Input: part model. Units: mm. Frame: model coordinates. A direction names the side the tool comes from. Coordinates: 2 decimals unless noted, no trailing zeros. Loops run counter-clockwise (first coordinate to the right, second up) from the corner with the lowest first, then second, coordinate; pieces in that order, holes last. Notation, with made-up numbers: (-7, -33.75) - (8, -33.75) arc R15 cw to (8, -4.75) - close; hole circle Ø5 at (-36, 87.25). An arc over 180 degrees is marked (long way). Use a Markdown table: item, result. Add a question column.
1. Draft query along Y for faces 1 (the face through (-9.43, -18.15, 2.03)), 2 (the face through (-5.56, 15.91, 2.03)), 3 (the face through (2, 0, 0)). Return one class per face: released by +Y, released by -Y, zero draft, split by the parting line, or undercut.
2. Section query B-B on y = -16. State how many separate pieces and enclosed holes the cut face has, then the cut area to 3 significant figures.
3. Ray query, L1, parallel to Z at x = 0.5, y = 0; L2, parallel to Y at x = 4.25, z = 0.25; L3, parallel to Y at x = 1, z = 2.8. Return the intervals inside material, ascending. Write a range as [from, to].
4. Access query for faces 4 (the face through (0, -0.3, 4.5)), 5 (the face through (5, 0, 5)), 6 (the face through (-3.173, -0.2, 1.5)). Directions: +Z, -Z, +X, -X, +Y, -Y. A direction counts if a zero-diameter tool reaches every point of the face in a straight line with its end or side. Return the directions, or none.
5. Section query A-A on y = -5. Return the cut outline in (x, z), then the cut area to 3 significant figures.
6. Contact query for flat-ended pins moving along their axis: P1, Ø0.8, axis at y = -3.5, z = 4.5, coming from the -X side; P2, Ø2, axis at y = -1, z = 2, coming from the -X side; P3, Ø11, axis at x = -6, y = 2.5, coming from the +Z side. Output: stop coordinate, or through.
```python
from build123d import *

# Parameters (mm, degrees)
F0_W      = 20
F0_H      = 37.5
F1_DEPTH  = 5
F2_W      = 10
F2_H      = 37.5
F3_DEPTH  = 1
F5_D      = 3
F6_W      = 6.8271449069
F6_H      = 23.5
F7_DEPTH  = 6
F8_R      = 2
F12_R     = 1.475
F13_DEPTH = 26
F16_R     = 1.475
F17_DEPTH = 27.5
F19_R     = 0.25
F20_DEPTH = 27.5


with BuildPart() as f1:
    # F0 (on Top) → F1 (new body)
    with BuildSketch(Plane.XY):
        Rectangle(F0_W, F0_H)
    extrude(amount=F1_DEPTH)

    # F2 (on face) → F3 (cut)
    with BuildSketch(Plane.XY.offset(5)):
        with Locations((-5, 0)):
            Rectangle(F2_W, F2_H)
    extrude(amount=-F3_DEPTH, mode=Mode.SUBTRACT)

    # F5 (through all)
    with Locations(Plane(origin=(0, 0, 0), x_dir=(1, 0, 0), z_dir=(0, 0, -1))):
        with Locations((-6.75, 15), (-6.75, -15)):
            Hole(F5_D / 2)

    # F6 (on Top) → F7 (cut)
    with BuildSketch(Plane.XY):
        with Locations((-6.5864275466, 0)):
            Rectangle(F6_W, F6_H)
    extrude(amount=F7_DEPTH, mode=Mode.SUBTRACT)

    # F8
    f8_edges = [f1.edges().sort_by_distance(p)[0] for p in [
        (-10, -18.75, 2),
        (10, -18.75, 2.5),
        (10, 18.75, 2.5),
        (-10, 18.75, 2),
        (-10, -11.75, 2),
        (-10, 11.75, 2),
    ]]
    fillet(f8_edges, radius=F8_R)

    # F12 (on line) → F13 (cut, symmetric)
    with BuildSketch(Plane(origin=(2.3968290702, -1.2522454416, 0), x_dir=(0.4630676024, 0.8863229635, 0), z_dir=(0.8863229635, -0.4630676024, 0))):
        with Locations((14.9191381368, 1.5)):
            Circle(F12_R)
    extrude(amount=F13_DEPTH, both=True, mode=Mode.SUBTRACT)

    # F16 (on line) → F17 (cut, symmetric)
    with BuildSketch(Plane(origin=(-0.5234543941, -0.2734835734, 0), x_dir=(-0.4630676024, 0.8863229635, 0), z_dir=(0.8863229635, 0.4630676024, 0))):
        with Locations((-14.9191381368, 1.5)):
            Circle(F16_R)
    extrude(amount=F17_DEPTH, both=True, mode=Mode.SUBTRACT)

    # F19 (on face) → F20 (cut, symmetric)
    with BuildSketch(Plane.YZ.offset(10)):
        with Locations((0, 2)):
            Circle(F19_R)
    extrude(amount=F20_DEPTH, both=True, mode=Mode.SUBTRACT)


solid = f1.part
```
Resolved:
| question | item | result |
|---|---|---|
| 1 | face 1 | released by -Y |
| 1 | face 2 | undercut |
| 1 | face 3 | zero draft |
| 2 | separate pieces | 2 |
| 2 | enclosed holes | 1 |
| 2 | area | 66.3 mm² |
| 3 | L1 | [0, 1.75], [2.25, 5] |
| 3 | L2 | [-18.75, -15.5], [-13.73, 13.73], [15.5, 18.75] |
| 3 | L3 | [-18.75, -17.1], [-15.52, 15.52], [17.1, 18.75] |
| 4 | face 4 | +Z, -X, +Y, -Y |
| 4 | face 5 | +Z, +X, -X, +Y, -Y |
| 4 | face 6 | +Z, -Z, -X |
| 5 | outline | (-3.17, 0) - (10, 0) - (10, 5) - (0, 5) - (0, 4) - (-3.17, 4) - close |
| 5 | area | 62.7 mm² |
| 6 | P1 | x = 0 |
| 6 | P2 | x = -3.17 |
| 6 | P3 | z = 4 |
